Input: part model. Units: mm. Frame: model coordinates. A direction names the side the tool comes from. Give positions to 0.01 mm unless a question says otherwise; leave off trailing zeros. Write each loop counter-clockwise with the first axis right and the second up, starting at its lowest first coordinate (ties: lowest second). Pieces come first, ordered by that corner, then holes. Notation, with made-up numbers: (49, -26.5) -> (83, -26.5) arc R29 cw to (83, 1.5) -> close; hole circle Ø6 at (83.25, -24). An arc over 180 degrees is marked (long way). Answer as a JSON object with one key per item and string values. Group by question number.
from build123d import *

# Parameters (mm, degrees)
SKETCH1_W           = 40
SKETCH1_H           = 18.5
SKETCH1_R           = 2.25
SKETCH1_H_2         = 1.5
BOSS_EXTRUDE3_DEPTH = 6
SKETCH1_5_R         = 1.75
BOSS_EXTRUDE4_DEPTH = 4
SKETCH2_R           = 2.5
SKETCH2_R_2         = 1.75
BOSS_EXTRUDE5_DEPTH = 1.5
SKETCH3_W           = 38
SKETCH3_H           = 18
CUT_EXTRUDE1_DEPTH  = 0.5


with BuildPart() as part:
    # Sketch1 → Boss-Extrude3 (new body)
    with BuildSketch(Plane(origin=(0, 0, 0), x_dir=(1, 0, 0), z_dir=(0, 1, 0))):
        with Locations((0, -0.75)):
            Rectangle(SKETCH1_W, SKETCH1_H)
        with Locations((-10, 0)):
            Circle(SKETCH1_R, mode=Mode.SUBTRACT)
        with Locations((10, 0)):
            Circle(SKETCH1_R, mode=Mode.SUBTRACT)
        with Locations((0, 10.75)):
            Rectangle(SKETCH1_W, SKETCH1_H_2)
        with Locations((0, 9.25)):
            Rectangle(SKETCH1_W, SKETCH1_H_2)
    extrude(amount=BOSS_EXTRUDE3_DEPTH)

    # Sketch1_5 → Boss-Extrude4 (add)
    with BuildSketch(Plane(origin=(0, 0, 0), x_dir=(1, 0, 0), z_dir=(0, 1, 0))):
        with BuildLine():
            Line((20, 11.5), (20, 10))
            Line((20, 10), (20, 8.5))
            ThreePointArc((20, 8.5), (32.5, 21), (20, 33.5))
            Line((20, 33.5), (3.708099244, 33.5))
            ThreePointArc((3.708099244, 33.5), (-4, 32), (3.708099244, 30.5))
            Line((3.708099244, 30.5), (20, 30.5))
            ThreePointArc((20, 30.5), (29.5, 21), (20, 11.5))
        make_face()
        with Locations((0, 32)):
            Circle(SKETCH1_5_R, mode=Mode.SUBTRACT)
    extrude(amount=BOSS_EXTRUDE4_DEPTH)

    # Sketch2 → Boss-Extrude5 (add)
    with BuildSketch(Plane(origin=(0, 4, 0), x_dir=(1, 0, 0), z_dir=(0, 1, 0))):
        with Locations((0, 32)):
            Circle(SKETCH2_R)
        with Locations((0, 32)):
            Circle(SKETCH2_R_2, mode=Mode.SUBTRACT)
    extrude(amount=BOSS_EXTRUDE5_DEPTH)

    # Sketch3 → Cut-Extrude1 (cut)
    with BuildSketch(Plane(origin=(0, 6, 0), x_dir=(1, 0, 0), z_dir=(0, 1, 0))):
        Rectangle(SKETCH3_W, SKETCH3_H)
    extrude(amount=-CUT_EXTRUDE1_DEPTH, mode=Mode.SUBTRACT)


solid = part.part
1. Mould query, pull axis X, two halves, no side actions, for faces 1 (the face through (-2, 6, -10)), 2 (the face through (20, 3, -1)), 3 (the face through (29.498, 1.972, -21.209)). Classes: pulls with the +X half, pulls with the -X half, needs draft (parallel to the pull), parting line crosses it, or undercut.
2. Section A-A (x = 15.5). Return the cut outline in (y, z).
3. Section B-B (z = 0). Return the cut outline in (x, y).
4. Reachability of faces 4 (the face through (0, 5.5, 0)), 5 (the face through (0, 3, -11.5)), 6 (the face through (12, 2, -33.5)), 7 (the face through (1, 5.5, -34)) from +Z, -Z, +X, -X, +Y, -Y: full face, straight path, thin tool, end or side. Return the list, or none.
5. Contact query for flat-ended pins moving along their axis: pin 1 Ø2.5 at (x, z) = (-10, 0) entering from -Y; pin 2 Ø22 at (x, z) = (11.5, -26) entering from +Y; pin 3 Ø3 at (x, y) = (-4.5, 5) entering from -Z; pin 4 Ø3 at (x, y) = (9.5, 3) entering from -Z. Output: stop coordinate, or through.
6. Section C-C (y = 3.1). Return the cut outline in (x, z), plus the area to 3 significant figures.
7. Line query: line 1 (Z direction, x = 10, y = 3.75); line 2 (Z direction, x = 0, y = 3.1); line 3 (X direction, y = 2.1, z = 0). Output: solid intervals per line, ascending.
8. Section D-D (x = 0). Return the cut outline in (y, z).
Working result:
{
 "1": {"face 1": "needs draft", "face 2": "pulls with the +X half", "face 3": "undercut"},
 "2": {"outline": "(0, -33.5) -> (4, -33.5) -> (4, -30.5) -> (0, -30.5) -> close; (0, -11.5) -> (6, -11.5) -> (6, -9) -> (5.5, -9) -> (5.5, 9) -> (6, 9) -> (6, 10) -> (0, 10) -> close"},
 "3": {"outline": "(-20, 0) -> (-12.25, 0) -> (-12.25, 5.5) -> (-19, 5.5) -> (-19, 6) -> (-20, 6) -> close; (-7.75, 0) -> (7.75, 0) -> (7.75, 5.5) -> (-7.75, 5.5) -> close; (12.25, 0) -> (20, 0) -> (20, 6) -> (19, 6) -> (19, 5.5) -> (12.25, 5.5) -> close"},
 "4": {"face 4": "+Y", "face 5": "-X, +Y, -Y", "face 6": "-Z, +X, +Y, -Y", "face 7": "-Z, +X, -X, +Y"},
 "5": {"pin 1": "passes through", "pin 2": "stops at y = 5.5", "pin 3": "stops at z = -34.14", "pin 4": "stops at z = -33.5"},
 "6": {"outline": "(-20, -11.5) -> (20, -11.5) arc R9.5 cw to (20, -30.5) -> (3.71, -30.5) arc R4 ccw (long way) to (3.71, -33.5) -> (20, -33.5) arc R12.5 ccw to (20, -8.5) -> (20, 10) -> (-20, 10) -> close; hole circle Ø4.5 at (-10, 0); hole circle Ø3.5 at (0, -32); hole circle Ø4.5 at (10, 0)", "area": "1,020 mm^2"},
 "7": {"line 1": "z = -33.5 to -30.5, -11.5 to -2.25, 2.25 to 10", "line 2": "z = -36 to -33.75, -30.25 to -28, -11.5 to 10", "line 3": "x = -20 to -12.25, -7.75 to 7.75, 12.25 to 20"},
 "8": {"outline": "(0, -36) -> (4, -36) -> (4, -34.5) -> (5.5, -34.5) -> (5.5, -33.75) -> (0, -33.75) -> close; (0, -30.25) -> (5.5, -30.25) -> (5.5, -29.5) -> (4, -29.5) -> (4, -28) -> (0, -28) -> close; (0, -11.5) -> (6, -11.5) -> (6, -9) -> (5.5, -9) -> (5.5, 9) -> (6, 9) -> (6, 10) -> (0, 10) -> close"}
}
